from build123d import *

# Parameters (mm, degrees)
SKETCH_1_W          = 63
SKETCH_1_H          = 58
EXTRUDE_1_DEPTH     = 1.6
SKETCH_2_R          = 1.65
CUT_EXTRUDE_1_DEPTH = 1.6
FILLET_1_R          = 3
SKETCH_3_R          = 1.65
CUT_EXTRUDE_2_DEPTH = 1.6


with BuildPart() as part:
    # 草图1 → 凸台-拉伸1 (new body)
    with BuildSketch(Plane(origin=(0, 0, 0), x_dir=(1, 0, 0), z_dir=(0, 1, 0))):
        Rectangle(SKETCH_1_W, SKETCH_1_H)
    extrude(amount=EXTRUDE_1_DEPTH)

    # 草图2 → 切除-拉伸1 (cut)
    with BuildSketch(Plane(origin=(0, 1.6, 0), x_dir=(1, 0, 0), z_dir=(0, 1, 0))):
        with Locations((-28.3, 25.75)):
            Circle(SKETCH_2_R)
        with Locations((28.3, 25.75)):
            Circle(SKETCH_2_R)
        with Locations((28.3, -25.75)):
            Circle(SKETCH_2_R)
        with Locations((-28.3, -25.75)):
            Circle(SKETCH_2_R)
    extrude(amount=-CUT_EXTRUDE_1_DEPTH, mode=Mode.SUBTRACT)

    # 圆角1
    fillet_1_edges = [part.edges().sort_by_distance(p)[0] for p in [
        (31.5, 0.8, 29),
        (-31.5, 0.8, 29),
        (-31.5, 0.8, -29),
        (31.5, 0.8, -29),
    ]]
    fillet(fillet_1_edges, radius=FILLET_1_R)

    # 草图3 → 切除-拉伸2 (cut)
    with BuildSketch(Plane(origin=(0, 1.6, 0), x_dir=(1, 0, 0), z_dir=(0, 1, 0))):
        with Locations((-28.3, 1.75)):
            Circle(SKETCH_3_R)
        with Locations((28.3, 1.75)):
            Circle(SKETCH_3_R)
    extrude(amount=-CUT_EXTRUDE_2_DEPTH, mode=Mode.SUBTRACT)


solid = part.part
The listing builds one solid part. Answer for the finished solid, in the listing's coordinates (mm). Give positions to 0.01 mm unless a question says otherwise; leave off trailing zeros. Write each loop counter-clockwise with the first axis right and the second up, starting at its lowest first coordinate (ties: lowest second). Pieces come first, ordered by that corner, then holes.
Item 1: Find the intervals of material crossed by line 1 along X through (y, z) = (0.85, 25.75); line 2 along Z through (x, y) = (28.3, 1.15); line 3 along X through (y, z) = (0.2, -25), in increasing order.
Item 2: Section B-B, the plane y = 1.35 is taken. Write down the section's boundary in (x, z).
Item 3: Determine the mould class of faces 1 (the cylindrical face through (-30.64, 0.81, -28.1)), 2 (the cylindrical face through (-29.516, 0.811, -26.865)), 3 (the flat face through (0, 1, 29)) for opening direction X: released by +X, released by -X, zero draft, split by the parting line, or undercut.
Item 4: Section A-A, the plane z = -1.75 is taken. Write down the section's boundary in (x, y), plus the area to 3 significant figures.
Completed:
1. line 1: x = -31.5 to -29.95, -26.65 to 26.65, 29.95 to 31.5
1. line 2: z = -29 to -27.4, -24.1 to -3.4, -0.1 to 24.1, 27.4 to 29
1. line 3: x = -31.5 to -29.77, -26.83 to 26.83, 29.77 to 31.5
2. outline: (-31.5, -26) arc R3 ccw to (-28.5, -29) - (28.5, -29) arc R3 ccw to (31.5, -26) - (31.5, 26) arc R3 ccw to (28.5, 29) - (-28.5, 29) arc R3 ccw to (-31.5, 26) - close; hole circle Ø3.3 at (-28.3, -25.75); hole circle Ø3.3 at (-28.3, -1.75); hole circle Ø3.3 at (-28.3, 25.75); hole circle Ø3.3 at (28.3, -25.75); hole circle Ø3.3 at (28.3, -1.75); hole circle Ø3.3 at (28.3, 25.75)
3. face 1: released by -X
3. face 2: undercut
3. face 3: zero draft
4. outline: (-31.5, 0) - (-29.95, 0) - (-29.95, 1.6) - (-31.5, 1.6) - close; (-26.65, 0) - (26.65, 0) - (26.65, 1.6) - (-26.65, 1.6) - close; (29.95, 0) - (31.5, 0) - (31.5, 1.6) - (29.95, 1.6) - close
4. area: 90.2 mm2
